Autodesk Inventor part; units mm, degrees
ref_plane "YZ Plane" through (0, 0, 0) normal (1, 0, 0) x (0, 1, 0)
ref_plane "XZ Plane" through (0, 0, 0) normal (0, 1, 0) x (-1, 0, 0)
ref_plane "XY Plane" through (0, 0, 0) normal (0, 0, 1) x (1, 0, 0)
sketch "Sketch1" plane through (0, 0, 0) normal (0, 0, 1) x (1, 0, 0)
  line L0 (0, 0) -> (278, 0)
  line L1 (278, 0) -> (278, 179)
  line L2 (278, 179) -> (0, 179)
  line L3 (0, 179) -> (0, 0)
  dimension "d0" = 278
  dimension "d1" = 179
extrude "Extrusion1" add sketch "Sketch1" along normal blind 3
sketch "Sketch2" plane through (0, 0, 3) normal (0, 0, 1) x (1, 0, 0)
  line L0 (0, 179) -> (0, 0)
  line L1 (278, 179) -> (0, 179)
  line L2 (278, 0) -> (278, 179)
  point P0 (20, 159)
  point P1 (258, 159)
  dimension "d4" = 20
  dimension "d5" = 20
  dimension "d6" = 20
  dimension "d7" = 20
hole "Hole1" at (20, 159, 3) at (258, 159, 3) direction (0, 0, -1) diameter 7 end through all
sketch "Sketch6" plane through (0, 179, 0) normal (0, 1, 0) x (1, 0, 0)
  line L0 (0, 0) -> (278, 0)
  line L1 (0, -3) -> (278, -3)
  line L2 (0, 0) -> (278, 0)
  line L3 (278, 0) -> (278, -3)
  line L4 (278, -3) -> (0, -3)
  line L5 (0, -3) -> (0, 0)
extrude "Extrusion2" add sketch "Sketch6" along normal blind 26
sketch "Sketch7" plane through (0, 0, 0) normal (0, 0, -1) x (-1, 0, 0)
  circle A0 centre (-92.17, 33.13) radius 1.5875
  circle A1 centre (-165.83, 33.13) radius 1.5875
  circle A2 centre (-166.592, 118.855) radius 1.5875
  circle A3 centre (-88.36, 118.855) radius 1.5875
  circle A4 centre (-8.5, 51.55) radius 1.6
  circle A5 centre (-72.5, 51.55) radius 1.6
  circle A6 centre (-72.5, 142.5) radius 1.6
  circle A7 centre (-8.5, 142.5) radius 1.6
  circle A8 centre (-86.6, 132.5) radius 1.6
  circle A9 centre (-86.6, 196.5) radius 1.6
  circle A10 centre (-177.55, 196.5) radius 1.6
  circle A11 centre (-177.55, 132.5) radius 1.6
  circle A12 centre (-184.55, 132.5) radius 1.6
  circle A13 centre (-184.55, 196.5) radius 1.6
  circle A14 centre (-275.5, 196.5) radius 1.6
  circle A15 centre (-275.5, 132.5) radius 1.6
  circle A16 centre (-275.5, 113.5) radius 1.6
  circle A17 centre (-275.5, 49.5) radius 1.6
  circle A18 centre (-184.55, 49.5) radius 1.6
  circle A19 centre (-184.55, 113.5) radius 1.6
  line L0 (0, 0) -> (-278, 0)
  line L1 (0, 0) -> (0, 205)
  line L2 (-278, 205) -> (0, 205)
  line L3 (-278, 0) -> (-278, 205)
  dimension "d41" = 33.13
  dimension "d42" = 51.55
  dimension "d43" = 51.55
  dimension "d44" = 8.5
  dimension "d45" = 72.5
  dimension "d46" = 88.36
  dimension "d47" = 92.17
  dimension "d48" = 165.83
  dimension "d49" = 166.592
  dimension "d50" = 86.6
  dimension "d51" = 177.55
  dimension "d52" = 8.5
  dimension "d53" = 72.5
  dimension "d54" = 2.5
  dimension "d55" = 93.45
  dimension "d56" = 91.5
  dimension "d57" = 155.5
  dimension "d58" = 118.855
properties part number "SupportsheetADCS2" material "Aluminum 6061"
Here's how the part is built. I have some questions about the finished solid (model axes, mm). Give positions to 0.01 mm unless a question says otherwise; leave off trailing zeros. Loops run counter-clockwise (first coordinate to the right, second up) from the corner with the lowest first, then second, coordinate; pieces in that order, holes last. Notation, with made-up numbers: M 27.5,-17 L 61.5,-17 A8 ccw 61.5,-10 Z; hole C 56.25,4 d9. An arc over 180 degrees is marked long. Use one line per item in the form item = value. Start each with the question number.
Q1. I need wall thicknesses on line 1 along X through (y, z) = (159, 1.35); line 2 along Y through (x, z) = (258, 1.7). Which ranges of each line are inside material? Lowest first, please.
Q2. Thinking about a two-plate mould opening in X: for faces 1 (the cylindrical face through (261.105, 157.385, 1.479)), 2 (the flat face through (137, 101, 0)), which applies, +X half, -X half, draft (parallel to the pull), parting line (faces both ways), or undercut?
Q3. If we section it at A-A (x = 20): Write out the boundary of the cut face in (y, z).
Q4. If we section it at B-B (y = 159): Write out the boundary of the cut face in (x, z), then the cut area to 3 significant figures.
Q5. Will this pin go through, and if not, where does the flat tip stop? pin 1 Ø8 at (x, y) = (258, 159) entering from +Z.
Taken from the geometry:
q1.line_1 = 0 to 16.5, 23.5 to 254.5, 261.5 to 278
q1.line_2 = 0 to 155.5, 162.5 to 205
q2.face_1 = undercut
q2.face_2 = draft
q3.outline = M 0,0 L 155.5,0 L 155.5,3 L 0,3 Z; M 162.5,0 L 205,0 L 205,3 L 162.5,3 Z
q4.outline = M 0,0 L 16.5,0 L 16.5,3 L 0,3 Z; M 23.5,0 L 254.5,0 L 254.5,3 L 23.5,3 Z; M 261.5,0 L 278,0 L 278,3 L 261.5,3 Z
q4.area = 792 mm^2
q5.pin_1 = 3
